```python
from build123d import *

# Parameters (mm, degrees)
SKETCH1_R           = 4.7625
BOSS_EXTRUDE1_DEPTH = 9.525
SKETCH2_R           = 38.1
BOSS_EXTRUDE2_DEPTH = 2.54
CUT_EXTRUDE1_DEPTH  = 55.716959208
CIRPATTERN1_COUNT   = 8


with BuildPart() as part:
    # Sketch1 → Boss-Extrude1 (new body)
    with BuildSketch(Plane(origin=(0, 0, 0), x_dir=(0, 0, -1), z_dir=(1, 0, 0))):
        with Locations(Location((0, 0, 0), (0, 0, 180))):
            Circle(SKETCH1_R)
        with BuildLine():
            Line((-1.905, -1.956171069), (-1.905, 1.956171069))
            ThreePointArc((-1.905, 1.956171069), (0, 2.7305), (1.905, 1.956171069))
            Line((1.905, 1.956171069), (1.905, -1.956171069))
            ThreePointArc((1.905, -1.956171069), (0, -2.7305), (-1.905, -1.956171069))
        make_face(mode=Mode.SUBTRACT)
    extrude(amount=BOSS_EXTRUDE1_DEPTH)

    # Sketch2 → Boss-Extrude2 (add)
    with BuildSketch(Plane.ZY):
        Circle(SKETCH2_R)
    extrude(amount=BOSS_EXTRUDE2_DEPTH)

    # Sketch3 → Cut-Extrude1 (cut, symmetric)
    with BuildSketch(Plane(origin=(0, 0, 0), x_dir=(0, 0, -1), z_dir=(1, 0, 0))):
        Polygon((-1.5875, 10.687130657), (0, 4.7625), (1.5875, 10.687130657), (1.5875, 38.1), (-1.5875, 38.1), align=None)
    cut_extrude1 = extrude(amount=CUT_EXTRUDE1_DEPTH, both=True, mode=Mode.SUBTRACT)

    # CirPattern1: Cut-Extrude1 ×8 about axis
    cirpattern1_axis = Axis((0, 0, 0), (1, 0, 0))
    for i in range(1, CIRPATTERN1_COUNT):
        add(cut_extrude1.rotate(cirpattern1_axis, i * 360 / CIRPATTERN1_COUNT), mode=Mode.SUBTRACT)


solid = part.part
```
Verification items for the finished model (mm, model axes). A direction names the side the tool comes from. Give positions to 0.01 mm unless a question says otherwise; leave off trailing zeros. Order: outer loops, then holes, each group sorted by start corner. A loop starts at its lowest first (then second) coordinate and runs counter-clockwise, first axis right, second up. Notation, with made-up numbers: (-27, 73.5) -> (16, 73.5) arc R30 cw to (16, 99.5) -> close; hole circle Ø3 at (50, -26). An arc over 180 degrees is marked (long way). Use a Markdown table: item, result.
1) Material ranges on probe 1 along Z at (x, y) = (-1, 17); probe 2 along Z at (x, y) = (-0.5, -3.5); probe 3 along X at (y, z) = (28, 6.5), recorded low to high.
Results:
| item | result |
|---|---|
| probe 1 | -34.1 to -19.25, -14.75 to -1.59, 1.59 to 14.75, 19.25 to 34.1 |
| probe 2 | -37.94 to -3.6, -3.44 to 3.44, 3.6 to 37.94 |
| probe 3 | -2.54 to 0 |
2) Mould release check, pull along Y, two halves, no side actions. Record for faces 4 (the cylindrical face through (-1.25, -14.41, -35.27)), 5 (the flat face through (-1, 24, -1.588)), 6 (the cylindrical face through (4.7, 4.65, -1.03)), 7 (the flat face through (-1.25, 0.78, 7.68)): pulls with the +Y half, pulls with the -Y half, needs draft (parallel to the pull), parting line crosses it, or undercut.
Results:
| item | result |
|---|---|
| face 4 | pulls with the -Y half |
| face 5 | needs draft |
| face 6 | parting line crosses it |
| face 7 | undercut |
3) Tool access check on faces 1 (the cylindrical face through (4.7, -2.73, -0.03)), 2 (the flat face through (-1.252, -15.979, 18.224)), 3 (the flat face through (-1, -1.588, -24)). Record the directions out of +Z, -Z, +X, -X, +Y, -Y that give a thin tool (end or side, any length) a straight path to the whole face; none if there is none.
Results:
| item | result |
|---|---|
| face 1 | +X |
| face 2 | +X, -X |
| face 3 | -Z, +X, -X |
4) Depth check by flat-ended pin: pin 1 Ø4 at (x, y) = (1, -7.5) entering from +Z; pin 2 Ø3 at (x, z) = (-1.5, -24) entering from -Y; pin 3 Ø1 at (y, z) = (18, -6) entering from +X. Enter the tip coordinate at first touch or a pass-through.
Results:
| item | result |
|---|---|
| pin 1 | z = 37.66 |
| pin 2 | y = -30.75 |
| pin 3 | x = 0 |
5) Section check B-B, the plane y = 16. Record the boundary of the cut face in (x, z).
Results:
| item | result |
|---|---|
| outline | (-2.54, -34.58) -> (0, -34.58) -> (0, -18.25) -> (-2.54, -18.25) -> close; (-2.54, -13.75) -> (0, -13.75) -> (0, -1.59) -> (-2.54, -1.59) -> close; (-2.54, 1.59) -> (0, 1.59) -> (0, 13.75) -> (-2.54, 13.75) -> close; (-2.54, 18.25) -> (0, 18.25) -> (0, 34.58) -> (-2.54, 34.58) -> close |
6) Section check A-A, the plane x = 6. Record the boundary of the cut face in (y, z) (1 decimal), then the cut area to 3 significant figures.
Results:
| item | result |
|---|---|
| outline | circle Ø9.5 at (0, 0); hole (-2, -1.9) -> (2, -1.9) arc R2.7 ccw to (2, 1.9) -> (-2, 1.9) arc R2.7 ccw to start |
| area | 52.3 mm² |
7) Section check C-C, the plane y = -17. Record the boundary of the cut face in (x, z), then the cut area to 3 significant figures.
Results:
| item | result |
|---|---|
| outline | (-2.54, -34.1) -> (0, -34.1) -> (0, -19.25) -> (-2.54, -19.25) -> close; (-2.54, -14.75) -> (0, -14.75) -> (0, -1.59) -> (-2.54, -1.59) -> close; (-2.54, 1.59) -> (0, 1.59) -> (0, 14.75) -> (-2.54, 14.75) -> close; (-2.54, 19.25) -> (0, 19.25) -> (0, 34.1) -> (-2.54, 34.1) -> close |
| area | 142 mm² |
